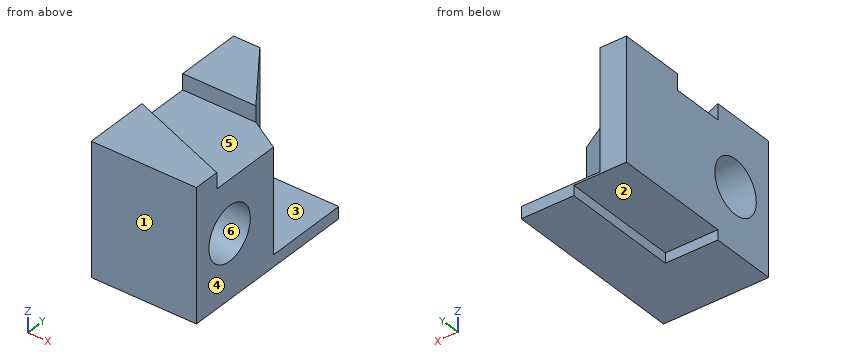
```python
from build123d import *

# Parameters (mm, degrees)
CROQUIS1_W              = 80
CROQUIS1_H              = 88
SALIENTE_EXTRUIR2_DEPTH = 50
SALIENTE_EXTRUIR3_DEPTH = 12
SALIENTE_EXTRUIR4_DEPTH = 90
SALIENTE_EXTRUIR5_DEPTH = 12
CORTAR_EXTRUIR1_DEPTH   = 79
CORTAR_EXTRUIR3_DEPTH   = 34
CROQUIS13_R             = 20.383603437
CORTAR_EXTRUIR5_DEPTH   = 80
SALIENTE_EXTRUIR8_DEPTH = 34
CORTAR_EXTRUIR7_DEPTH   = 79


with BuildPart() as part:
    # Croquis1 → Saliente-Extruir2 (new body)
    with BuildSketch(Plane(origin=(0, 0, 0), x_dir=(1, 0, 0), z_dir=(0, 1, 0))):
        Rectangle(CROQUIS1_W, CROQUIS1_H)
    extrude(amount=SALIENTE_EXTRUIR2_DEPTH)

    # Croquis3 → Saliente-Extruir3 (add)
    with BuildSketch(Plane.XY.offset(44)):
        Polygon((40, 0), (40, 20), (-40, 50), (-40, 0), align=None)
    extrude(amount=SALIENTE_EXTRUIR3_DEPTH)

    # Croquis4 → Saliente-Extruir4 (add)
    with BuildSketch(Plane(origin=(0, 50, 0), x_dir=(1, 0, 0), z_dir=(0, 1, 0))):
        Polygon((-40, -44), (-40, 36.464593772), (-20, 36.464593772), (0, 36.464593772), (0, 44), (40, 44), (40, -44), align=None)
    extrude(amount=SALIENTE_EXTRUIR4_DEPTH)

    # Croquis6 → Saliente-Extruir5 (add)
    with BuildSketch(Plane.XY.offset(44)):
        Polygon((-40, 140), (-40, 90), (15.619160928, 90), (-20.00024501, 140), align=None)
    extrude(amount=SALIENTE_EXTRUIR5_DEPTH)

    # Croquis7 → Cortar-Extruir1 (cut)
    with BuildSketch(Plane.XY.offset(44)):
        Polygon((-20.00024501, 140), (40, 140), (40, 90), (15.619160928, 90), align=None)
    extrude(amount=-CORTAR_EXTRUIR1_DEPTH, mode=Mode.SUBTRACT)

    # Croquis8 → Cortar-Extruir3 (cut)
    with BuildSketch(Plane(origin=(40, 0, 0), x_dir=(0, 0, -1), z_dir=(1, 0, 0))):
        Polygon((35, 90), (35, 61.907696256), (-44, 60.140404664), (-44, 90), align=None)
    extrude(amount=-CORTAR_EXTRUIR3_DEPTH, mode=Mode.SUBTRACT)

    # Croquis13 → Cortar-Extruir5 (cut)
    with BuildSketch(Plane(origin=(40, 0, 0), x_dir=(0, 0, -1), z_dir=(1, 0, 0))):
        with Locations((-4.438083907, 32.611633529)):
            Circle(CROQUIS13_R)
    extrude(amount=-CORTAR_EXTRUIR5_DEPTH, mode=Mode.SUBTRACT)

    # Croquis16 → Saliente-Extruir8 (add)
    with BuildSketch(Plane(origin=(6, 0, 0), x_dir=(0, 0, -1), z_dir=(1, 0, 0))):
        Polygon((-44, 90), (35, 90), (35, 61.907696256), (-44, 60.140404664), align=None)
    extrude(amount=SALIENTE_EXTRUIR8_DEPTH)

    # Croquis17 → Cortar-Extruir7 (cut)
    with BuildSketch(Plane.XY.offset(44)):
        Polygon((15.619160928, 90), (40, 75.759565592), (40, 90), align=None)
    extrude(amount=-CORTAR_EXTRUIR7_DEPTH, mode=Mode.SUBTRACT)


solid = part.part
```
Could you check a few things on this model? Use its own coordinates, in mm. Face numbers are marked on the shaded views. A direction names the side the tool comes from. Coordinates: 2 decimals unless noted, no trailing zeros. Loops run counter-clockwise (first coordinate to the right, second up) from the corner with the lowest first, then second, coordinate; pieces in that order, holes last.
1) Imagine slicing it at A-A (z = -5.5). List the corners of the cut face in (x, y) for me, and give its area (3 significant figures).
Reported:
outline: (-40, 0) - (40, 0) - (40, 14.81) - (-40, 14.81) - close; (-40, 50.41) - (40, 50.41) - (40, 75.76) - (15.62, 90) - (-20, 140) - (-40, 140) - close
area: 6,070 mm2
2) Will these pins go through, and if not, where does the flat tip stop? pin 1 Ø10 at (y, z) = (112, -22.5) entering from +X; pin 2 Ø4 at (y, z) = (107.5, -40) entering from -X; pin 3 Ø1.5 at (x, y) = (-26, 120.5) entering from -Z.
Reported:
pin 1: stops at x = 3.51
pin 2: stops at x = 0
pin 3: stops at z = -36.46
3) Imagine slicing it at B-B (x = 22.5). List the corners of the cut face in (y, z) for me, and give its area (3 significant figures).
Reported:
outline: (0, -44) - (140, -44) - (140, -35) - (85.98, -35) - (85.98, 44) - (26.56, 44) - (26.56, 56) - (0, 56) - close; hole circle Ø40.77 at (32.61, 4.44)
area: 7,070 mm2
4) Imagine slicing it at D-D (z = -30.5). List the corners of the cut face in (x, y) for me.
Reported:
outline: (-40, 0) - (40, 0) - (40, 75.76) - (15.62, 90) - (-20, 140) - (-40, 140) - close
5) Please list where these lines run through material, in increasing order: line 1 along Z through (x, y) = (23, 64); line 2 along Z through (x, y) = (-27, 69); line 3 along Y through (x, z) = (23, 7.5).
Reported:
line 1: z = -44 to 44
line 2: z = -36.46 to 44
line 3: y = 0 to 12.46, 52.76 to 85.69
6) Imagine slicing it at C-C (y = 18). List the corners of the cut face in (x, z) for me, and give its area (3 significant figures).
Reported:
outline: (-40, -44) - (40, -44) - (40, -9.77) - (-40, -9.77) - close; (-40, 18.65) - (40, 18.65) - (40, 56) - (-40, 56) - close
area: 5,730 mm2
7) Which directions (+Z, -Z, +X, -X, +Y, -Y) give clear straight access to the entire face, cutting with the end or side of a thin tool? Please do the marked faces 1, 2 and 3.
Reported:
face 1: +Z, -Z, +X, -X, -Y
face 2: -Z, -X, +Y
face 3: +Z, +X, +Y
8) Thinking about a two-plate mould opening in Z: for the marked faces 4, 5 and 6, which applies, released by +Z, released by -Z, zero draft, split by the parting line, or undercut?
Reported:
face 4: zero draft
face 5: released by +Z
face 6: undercut
